Verification items for the finished model (mm, model axes). Face numbers are marked on the shaded views. A direction names the side the tool comes from. Coordinates: 2 decimals unless noted, no trailing zeros. Write each loop counter-clockwise with the first axis right and the second up, starting at its lowest first coordinate (ties: lowest second). Pieces come first, ordered by that corner, then holes. Notation, with made-up numbers: M 30,-9 L 69,-9 A30 cw 69,18 Z; hole C 48.25,18 d3. An arc over 180 degrees is marked long. One line per item, written item: value.
```python
from build123d import *

# Parameters (mm, degrees)
SKETCH_1_R          = 11
EXTRUDE_1_DEPTH     = 9
SKETCH_2_R          = 0.5
CUT_EXTRUDE_1_DEPTH = 18.972200756
SKETCH_3_R          = 16.549134696
SKETCH_3_R_2        = 9.25
CUT_EXTRUDE_2_DEPTH = 7
SKETCH_4_W          = 2
SKETCH_4_H          = 1.7
SKETCH_5_W          = 5
SKETCH_5_H          = 6
CUT_EXTRUDE_3_DEPTH = 7
SKETCH_6_R          = 1.4
CUT_EXTRUDE_4_DEPTH = 7
SKETCH_7_R          = 1.25
CUT_EXTRUDE_5_DEPTH = 2.5
CUT_EXTRUDE_START   = -1.5
SKETCH_8_R          = 1.25
CUT_EXTRUDE_6_DEPTH = 1.5
SKETCH_9_W          = 7
SKETCH_9_H          = 8
SKETCH_9_W_2        = 5
SKETCH_9_H_2        = 6
CUT_EXTRUDE_7_DEPTH = 2
CHAMFER_1_SIZE      = 0.5


with BuildPart() as part:
    # 草图1 → 凸台-拉伸1 (new body)
    with BuildSketch(Plane(origin=(0, 0, 0), x_dir=(1, 0, 0), z_dir=(0, 1, 0))):
        with Locations(Location((0, 0, 0), (0, 0, 270))):
            Circle(SKETCH_1_R)
    extrude(amount=EXTRUDE_1_DEPTH)

    # 草图2 → 切除-拉伸1 (cut, through all)
    with BuildSketch(Plane(origin=(0, 9, 0), x_dir=(1, 0, 0), z_dir=(0, 1, 0))):
        with Locations(Location((-5.5, 0, 0), (0, 0, 270))):
            Circle(SKETCH_2_R)
        with Locations(Location((5.5, 0, 0), (0, 0, 270))):
            Circle(SKETCH_2_R)
    extrude(amount=-CUT_EXTRUDE_1_DEPTH, mode=Mode.SUBTRACT)

    # 草图3 → 切除-拉伸2 (cut)
    with BuildSketch(Plane.XZ):
        Circle(SKETCH_3_R)
        with Locations(Location((0, 0, 0), (0, 0, 270))):
            Circle(SKETCH_3_R_2, mode=Mode.SUBTRACT)
    extrude(amount=-CUT_EXTRUDE_2_DEPTH, mode=Mode.SUBTRACT)

    # 草图4 → 切除-旋转1 (revolve, cut)
    with BuildSketch(Plane.XY, mode=Mode.PRIVATE) as cut_revolve_1_sk:
        with Locations((-9.25, 5.45)):
            Rectangle(SKETCH_4_W, SKETCH_4_H)
        with Locations((-9.25, 2.35)):
            Rectangle(SKETCH_4_W, SKETCH_4_H)
    revolve(cut_revolve_1_sk.sketch.rotate(Axis((0, 0, 0), (0, 1, 0)), 270), axis=Axis((0, 0, 0), (0, 1, 0)), mode=Mode.SUBTRACT)

    # 草图5 → 切除-拉伸3 (cut)
    with BuildSketch(Plane.XZ):
        Rectangle(SKETCH_5_W, SKETCH_5_H)
    extrude(amount=-CUT_EXTRUDE_3_DEPTH, mode=Mode.SUBTRACT)

    # 草图6 → 切除-拉伸4 (cut)
    with BuildSketch(Plane(origin=(0, 9, 0), x_dir=(1, 0, 0), z_dir=(0, 1, 0))):
        with Locations(Location((0, 0, 0), (0, 0, 270))):
            Circle(SKETCH_6_R)
    extrude(amount=-CUT_EXTRUDE_4_DEPTH, mode=Mode.SUBTRACT)

    # 草图7 → 切除-拉伸5 (cut)
    with BuildSketch(Plane(origin=(0, 9, 0), x_dir=(1, 0, 0), z_dir=(0, 1, 0))):
        with Locations(Location((-5.5, 0, 0), (0, 0, 270))):
            Circle(SKETCH_7_R)
        with Locations(Location((5.5, 0, 0), (0, 0, 270))):
            Circle(SKETCH_7_R)
    extrude(amount=-CUT_EXTRUDE_5_DEPTH, mode=Mode.SUBTRACT)

    # 草图8 → 切除-拉伸6 (cut)
    with BuildSketch(Plane.XZ.offset(CUT_EXTRUDE_START)):
        with Locations(Location((-5.5, 0, 0), (0, 0, 90))):
            Circle(SKETCH_8_R)
        with Locations(Location((5.5, 0, 0), (0, 0, 90))):
            Circle(SKETCH_8_R)
    extrude(amount=CUT_EXTRUDE_6_DEPTH, mode=Mode.SUBTRACT)

    # 草图9 → 切除-拉伸7 (cut)
    with BuildSketch(Plane.XZ):
        Rectangle(SKETCH_9_W, SKETCH_9_H)
        Rectangle(SKETCH_9_W_2, SKETCH_9_H_2, mode=Mode.SUBTRACT)
    extrude(amount=-CUT_EXTRUDE_7_DEPTH, mode=Mode.SUBTRACT)

    # 倒角1
    chamfer_1_edges = [part.edges().sort_by_distance(p)[0] for p in [
        (0, 0, 9.25),
    ]]
    chamfer(chamfer_1_edges, length=CHAMFER_1_SIZE)


solid = part.part
```
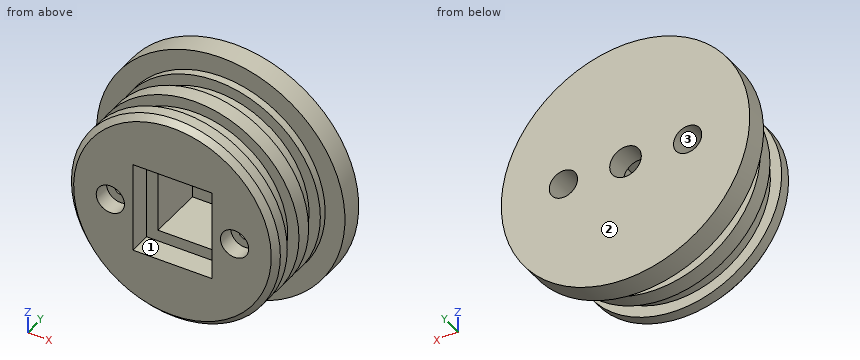
Item 1: Go/stop test with flat-tipped pins: P1, Ø2, axis at x = 5.5, z = 0, coming from the -Y side; P2, Ø5, axis at y = 3, z = 0.5, coming from the +X side; P3, Ø1.5, axis at x = 0.5, z = -0.5, coming from the -Y side. Record where each tip stops, or that it passes through.
The answers:
P1: stops at y = 1.5
P2: stops at x = 9.25
P3: stops at y = 7
Item 2: Cross-section at C-C, the plane y = 5.75. Enter the section's corners in (x, z), and give its area (3 significant figures).
The answers:
outline: C 0,0 d16.5; hole C -5.5,0 d1; hole M -2.5,-3 L 2.5,-3 L 2.5,3 L -2.5,3 Z; hole C 5.5,0 d1
area: 182 mm²
Item 3: Cross-section at A-A, the plane y = 1. Enter the section's corners in (x, z), and give its area (3 significant figures).
The answers:
outline: C 0,0 d18.5; hole C -5.5,0 d2.5; hole M -3.5,-4 L 3.5,-4 L 3.5,4 L -3.5,4 Z; hole C 5.5,0 d2.5
area: 203 mm²
Item 4: Cross-section at B-B, the plane z = 0. Give the number of separate pieces and of enclosed holes in the cut face, and give its area (4 significant figures).
The answers:
separate pieces: 4
enclosed holes: 0
area: 91.85 mm²
Item 5: Scan lines: line 1 (X direction, y = 8.25, z = 0); line 2 (X direction, y = 4.9, z = 0); line 3 (Y direction, x = 0.25, z = -9). Record each from-to range of solid material in increasing order.
The answers:
line 1: x = -11 to -6.75, -4.25 to -1.4, 1.4 to 4.25, 6.75 to 11
line 2: x = -8.25 to -6, -5 to -2.5, 2.5 to 5, 6 to 8.25
line 3: y = 0.25 to 1.5, 3.2 to 4.6, 6.3 to 9
Item 6: Access from +Z, -Z, +X, -X, +Y, -Y to the whole of each face (thin tool, end or side, straight path). Record for the marked faces 1, 2 and 3.
The answers:
face 1: -Y
face 2: +Z, -Z, +X, -X, +Y
face 3: +Y
